The drawing under review shows one solid part. Ordinate dimensions are in mm from its lowest x, y, z. A direction names the side the tool comes from. Give positions to 0.01 mm unless a question says otherwise; leave off trailing zeros. Write each loop counter-clockwise with the first axis right and the second up, starting at its lowest first coordinate (ties: lowest second). Pieces come first, ordered by that corner, then holes.
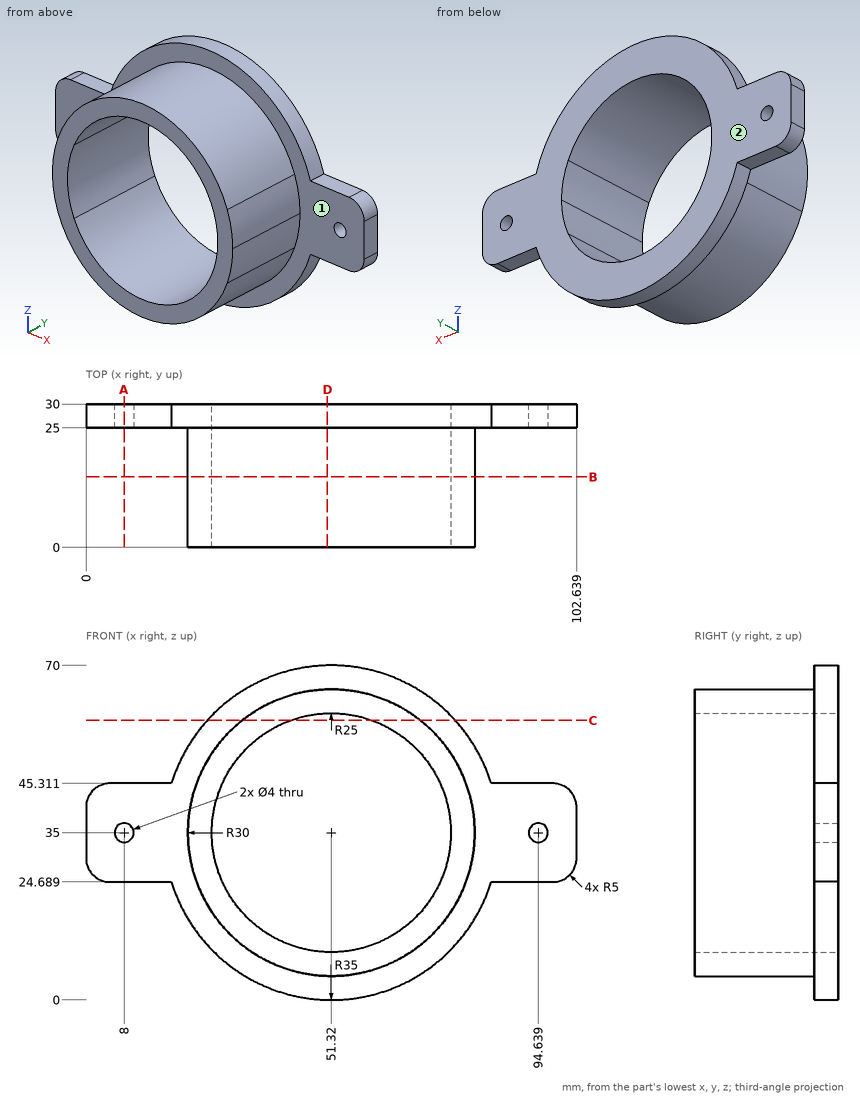
1) To check wall thickness, follow probe 1 along Z at (x, y) = (8, 27.1); probe 2 along Z at (x, y) = (52, 6.75); probe 3 along Y at (x, z) = (65.5, 8.5). State the ranges of each line that lie inside material, in increasing order.
2) Consider section C-C, the plane z = 58.5. Give the boundary of the cut face in (x, y).
3) Tool access review of the marked faces 1 and 2: name each direction out of +Z, -Z, +X, -X, +Y, -Y from which nothing blocks a thin tool from reaching the whole face with its end or side.
4) Consider section B-B, the plane y = 14.75. Give the boundary of the cut face in (x, z) (1 decimal), then the cut area to 3 significant figures.
5) Consider section A-A, the plane x = 8. Give the boundary of the cut face in (y, z).
6) Insertion check: pin 1 (4 mm diameter, centred on x = 14.5, y = 28, fed in from -Z); pin 2 (4 mm diameter, centred on x = 10, y = 27, fed in from +Z); pin 3 (10 mm diameter, centred on y = 16, z = 29, fed in from -X). Each pin has a flat end and moves straight along its axis. Give the tip position at first contact, or say it passes through.
7) Consider section D-D, the plane x = 50.5. Give the boundary of the cut face in (y, z), then the cut area to 3 significant figures.
Answer block:
1. probe 1: z = 24.69 to 33, 37 to 45.31
1. probe 2: z = 5.01 to 10.01, 59.99 to 64.99
1. probe 3: y = 25 to 30
2. outline: (25.38, 25) - (32.67, 25) - (32.67, 0) - (42.79, 0) - (42.79, 30) - (25.38, 30) - close; (59.85, 0) - (69.97, 0) - (69.97, 25) - (77.26, 25) - (77.26, 30) - (59.85, 30) - close
3. face 1: -Y
3. face 2: +Z, -Z, +X, -X, +Y
4. outline: circle Ø60 at (51.3, 35); hole circle Ø50 at (51.3, 35)
4. area: 864 mm2
5. outline: (25, 24.69) - (30, 24.69) - (30, 33) - (25, 33) - close; (25, 37) - (30, 37) - (30, 45.31) - (25, 45.31) - close
6. pin 1: stops at z = 24.69
6. pin 2: stops at z = 45.31
6. pin 3: stops at x = 21.34
7. outline: (0, 5.01) - (25, 5.01) - (25, 0.01) - (30, 0.01) - (30, 10.01) - (0, 10.01) - close; (0, 59.99) - (30, 59.99) - (30, 69.99) - (25, 69.99) - (25, 64.99) - (0, 64.99) - close
7. area: 350 mm2
